```python
from build123d import *

# Parameters (mm, degrees)
SKETCH3_W           = 125
SKETCH3_H           = 205
BOSS_EXTRUDE1_DEPTH = 6
SKETCH4_W           = 15
SKETCH4_H           = 50
SKETCH4_W_2         = 50
SKETCH4_H_2         = 15
CUT_EXTRUDE1_DEPTH  = 6
SKETCH5_W           = 12
SKETCH5_H           = 6
SKETCH5_W_2         = 6
SKETCH5_H_2         = 12
BOSS_EXTRUDE2_DEPTH = 6


with BuildPart() as part:
    # Sketch3 → Boss-Extrude1 (new body)
    with BuildSketch(Plane(origin=(0, 0, 0), x_dir=(1, 0, 0), z_dir=(0, 1, 0))):
        Rectangle(SKETCH3_W, SKETCH3_H)
    extrude(amount=BOSS_EXTRUDE1_DEPTH)

    # Sketch4 → Cut-Extrude1 (cut)
    with BuildSketch(Plane(origin=(0, 6, 0), x_dir=(1, 0, 0), z_dir=(0, 1, 0))):
        with Locations((-40, 40)):
            Rectangle(SKETCH4_W, SKETCH4_H)
        with Locations((40, 40)):
            Rectangle(SKETCH4_W, SKETCH4_H)
        Rectangle(SKETCH4_W_2, SKETCH4_H_2)
        with Locations((-40, -40)):
            Rectangle(SKETCH4_W, SKETCH4_H)
        with Locations((40, -40)):
            Rectangle(SKETCH4_W, SKETCH4_H)
        with Locations((0, 80)):
            Rectangle(SKETCH4_W_2, SKETCH4_H_2)
        with Locations((0, -80)):
            Rectangle(SKETCH4_W_2, SKETCH4_H_2)
    extrude(amount=-CUT_EXTRUDE1_DEPTH, mode=Mode.SUBTRACT)

    # Sketch5 → Boss-Extrude2 (add)
    with BuildSketch(Plane(origin=(0, 6, 0), x_dir=(1, 0, 0), z_dir=(0, 1, 0))):
        with Locations((24, -105.5)):
            Rectangle(SKETCH5_W, SKETCH5_H)
        with Locations((0, -105.5)):
            Rectangle(SKETCH5_W, SKETCH5_H)
        with Locations((-65.5, -84)):
            Rectangle(SKETCH5_W_2, SKETCH5_H_2)
        with Locations((-65.5, -60)):
            Rectangle(SKETCH5_W_2, SKETCH5_H_2)
        with Locations((-65.5, -12)):
            Rectangle(SKETCH5_W_2, SKETCH5_H_2)
        with Locations((65.5, -84)):
            Rectangle(SKETCH5_W_2, SKETCH5_H_2)
        with Locations((65.5, -36)):
            Rectangle(SKETCH5_W_2, SKETCH5_H_2)
        with Locations((65.5, -12)):
            Rectangle(SKETCH5_W_2, SKETCH5_H_2)
        with Locations((65.5, 12)):
            Rectangle(SKETCH5_W_2, SKETCH5_H_2)
        with Locations((65.5, 36)):
            Rectangle(SKETCH5_W_2, SKETCH5_H_2)
        with Locations((65.5, 84)):
            Rectangle(SKETCH5_W_2, SKETCH5_H_2)
        with Locations((24, 105.5)):
            Rectangle(SKETCH5_W, SKETCH5_H)
        with Locations((0, 105.5)):
            Rectangle(SKETCH5_W, SKETCH5_H)
        with Locations((-24, 105.5)):
            Rectangle(SKETCH5_W, SKETCH5_H)
        with Locations((-48, 105.5)):
            Rectangle(SKETCH5_W, SKETCH5_H)
        with Locations((-65.5, 36)):
            Rectangle(SKETCH5_W_2, SKETCH5_H_2)
        with Locations((-65.5, 12)):
            Rectangle(SKETCH5_W_2, SKETCH5_H_2)
        with Locations((48, -105.5)):
            Rectangle(SKETCH5_W, SKETCH5_H)
        with Locations((-24, -105.5)):
            Rectangle(SKETCH5_W, SKETCH5_H)
        with Locations((-48, -105.5)):
            Rectangle(SKETCH5_W, SKETCH5_H)
        with Locations((-65.5, -36)):
            Rectangle(SKETCH5_W_2, SKETCH5_H_2)
        with Locations((65.5, -60)):
            Rectangle(SKETCH5_W_2, SKETCH5_H_2)
        with Locations((65.5, 60)):
            Rectangle(SKETCH5_W_2, SKETCH5_H_2)
        with Locations((48, 105.5)):
            Rectangle(SKETCH5_W, SKETCH5_H)
        with Locations((-65.5, 84)):
            Rectangle(SKETCH5_W_2, SKETCH5_H_2)
        with Locations((-65.5, 60)):
            Rectangle(SKETCH5_W_2, SKETCH5_H_2)
    extrude(amount=-BOSS_EXTRUDE2_DEPTH)


solid = part.part
```
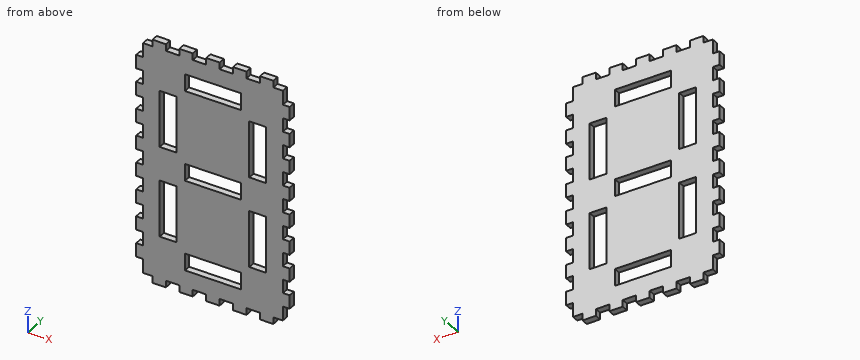
Here's how the part is built. I have some questions about the finished solid (model axes, mm). Coordinates: 2 decimals unless noted, no trailing zeros. Order: outer loops, then holes, each group sorted by start corner. A loop starts at its lowest first (then second) coordinate and runs counter-clockwise, first axis right, second up. Notation, with made-up numbers: M 46.5,47 L 69.5,47 A12 cw 69.5,60 Z; hole C -24.5,-31.5 d3. An arc over 180 degrees is marked long. Answer as a JSON object with one key per item and string values. Group by question number.
(1) I need wall thicknesses on probe 1 along Z at (x, y) = (-33, 4); probe 2 along Z at (x, y) = (-43.5, 4.7); probe 3 along X at (y, z) = (5.55, 53.5). Which ranges of each line are inside material? Lowest first, please.
(2) Suppose I cut it at B-B, the plane x = 12. Please give me the cut outline in (y, z).
(3) For pin 1 (3 mm diameter, centred on x = 65, y = 2.5, fed in from -Z); pin 2 (3 mm diameter, centred on y = 3, z = -106, fed in from -X); pin 3 (1.8 mm diameter, centred on y = 2, z = -77, fed in from -X), each with a flat end and sliding along its axis, tell me the tip position at first contact or that it passes through.
(4) Suppose I cut it at A-A, the plane z = -1.5. Please give me the cut outline in (x, y), then the cut area to 3 significant figures.
(5) Suppose I cut it at C-C, the plane z = -48. Please give me the cut outline in (x, y).
(6) Suppose I cut it at D-D, the plane z = -83. Please give me the cut outline in (x, y), then the cut area to 3 significant figures.
Values found:
{
 "1": {"probe 1": "z = -102.5 to -65, -15 to 15, 65 to 102.5", "probe 2": "z = -108.5 to -65, -15 to 15, 65 to 108.5", "probe 3": "x = -62.5 to -47.5, -32.5 to 32.5, 47.5 to 62.5"},
 "2": {"outline": "M 0,-102.5 L 6,-102.5 L 6,-87.5 L 0,-87.5 Z; M 0,-72.5 L 6,-72.5 L 6,-7.5 L 0,-7.5 Z; M 0,7.5 L 6,7.5 L 6,72.5 L 0,72.5 Z; M 0,87.5 L 6,87.5 L 6,102.5 L 0,102.5 Z"},
 "3": {"pin 1": "stops at z = -90", "pin 2": "stops at x = -54", "pin 3": "stops at x = -62.5"},
 "4": {"outline": "M -62.5,0 L -25,0 L -25,6 L -62.5,6 Z; M 25,0 L 62.5,0 L 62.5,6 L 25,6 Z", "area": "450 mm^2"},
 "5": {"outline": "M -62.5,0 L -47.5,0 L -47.5,6 L -62.5,6 Z; M -32.5,0 L 32.5,0 L 32.5,6 L -32.5,6 Z; M 47.5,0 L 62.5,0 L 62.5,6 L 47.5,6 Z"},
 "6": {"outline": "M -68.5,0 L -25,0 L -25,6 L -68.5,6 Z; M 25,0 L 68.5,0 L 68.5,6 L 25,6 Z", "area": "522 mm^2"}
}
